Work out the finished part from the listing and answer in its coordinate system (mm). Coordinates: 2 decimals unless noted, no trailing zeros. Order: outer loops, then holes, each group sorted by start corner. A loop starts at its lowest first (then second) coordinate and runs counter-clockwise, first axis right, second up. Notation, with made-up numbers: M 76.5,42 L 135.5,42 A21 cw 135.5,81 Z; hole C 34,57 d4. An arc over 180 degrees is marked long. Use a Markdown table: item, result.
Autodesk Inventor part; units mm, degrees
ref_plane "YZ Plane" through (0, 0, 0) normal (1, 0, 0) x (0, 1, 0)
ref_plane "XZ Plane" through (0, 0, 0) normal (0, 1, 0) x (-1, 0, 0)
ref_plane "XY Plane" through (0, 0, 0) normal (0, 0, 1) x (1, 0, 0)
sketch "Sketch1" plane through (0, 0, 0) normal (0, 0, 1) x (1, 0, 0)
  line L0 (150, -15) -> (-150, -15)
  line L1 (-150, -15) -> (-150, 15)
  line L2 (-150, 15) -> (150, 15)
  line L3 (150, 15) -> (150, -15)
  line L4 (150, -15) -> (-150, 15) construction
  line L5 (-150, -15) -> (150, 15) construction
  point P0 (0, 0)
  dimension "d0" = 300
  dimension "d1" = 30
extrude "Extrusion1" add sketch "Sketch1" along normal blind 10
chamfer "Chamfer1" distance 10 angle 45 1 edges at (0, 15, 10)
thicken "Thicken1" operation add thickness 20 both sides no extend neighbours yes toward (0, -1, 0) faces at (-50, -15, 3.3333)
properties part number "ball_ramp"
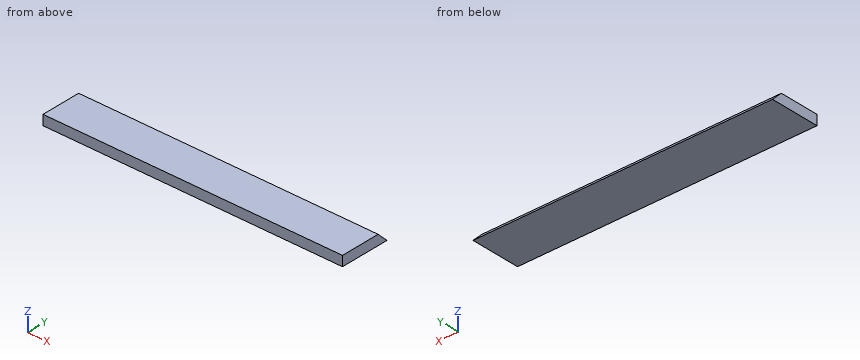
(1) A cutting plane is placed at C-C (y = 12). Determine the outline of the cut face in (x, z).
Conclusion:
| item | result |
|---|---|
| outline | M -150,0 L 150,0 L 150,3 L -150,3 Z |
(2) A cutting plane is placed at B-B (z = 4). Determine the outline of the cut face in (x, y).
Conclusion:
| item | result |
|---|---|
| outline | M -150,-35 L 150,-35 L 150,11 L -150,11 Z |
(3) Straight lines are drawn through the part: L1, parallel to Y at x = 23.5, z = 5; L2, parallel to Z at x = -134.5, y = 6; L3, parallel to Y at x = -42, z = 8.75. For each, find the intervals that lie inside material, in ascending order.
Conclusion:
| item | result |
|---|---|
| L1 | -35 to 10 |
| L2 | 0 to 9 |
| L3 | -35 to 6.25 |
